Part print with two shaded views. Sizes in mm from the minimum x, y, z corner. A direction names the side the tool comes from. Round coordinates to 2 decimals unless told otherwise and drop trailing zeros. Write each loop counter-clockwise with the first axis right and the second up, starting at its lowest first coordinate (ties: lowest second). Pieces come first, ordered by that corner, then holes. Notation, with made-up numbers: (0, 78.5) -> (25, 78.5) arc R20 cw to (25, 108.5) -> close; hole circle Ø10 at (-27, 40). An arc over 180 degrees is marked (long way). Answer as CSV lines item,"result".
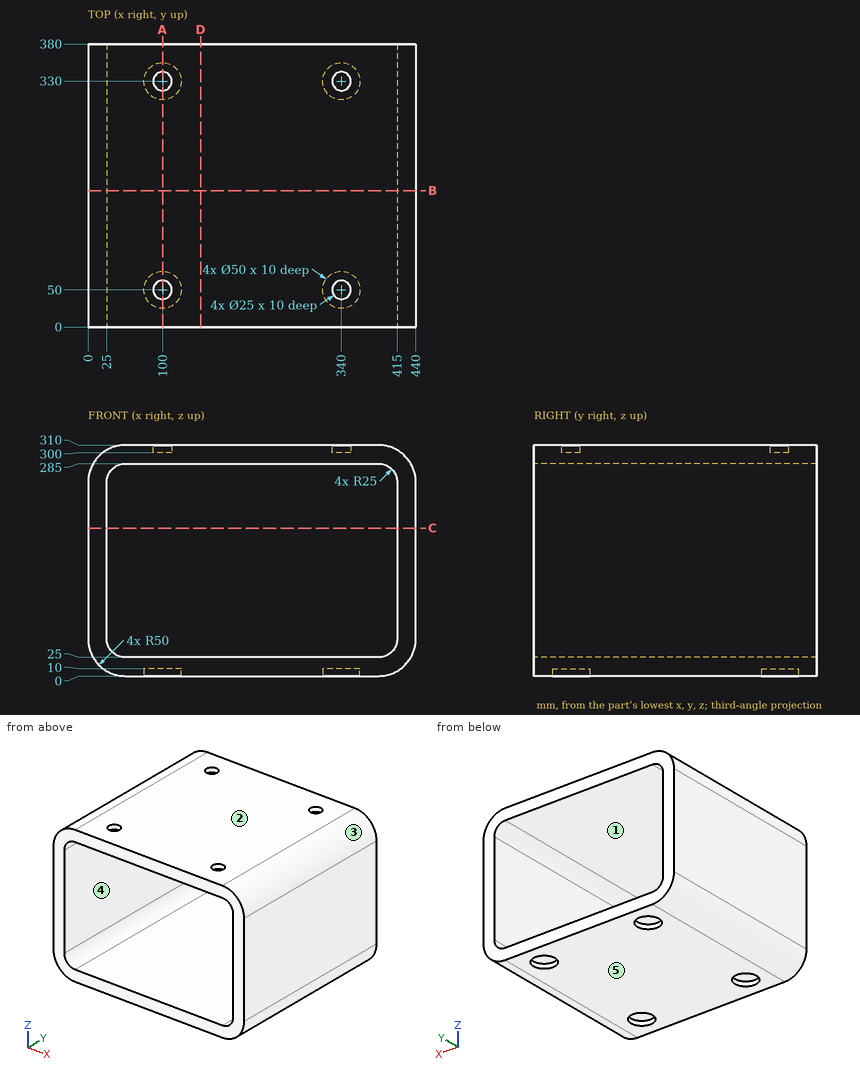
1. Cut at C-C, the plane z = 198.5. Write the cut outline in (x, y), then the cut area to 3 significant figures.
Results found:
outline,"(0, 0) -> (25, 0) -> (25, 380) -> (0, 380) -> close; (415, 0) -> (440, 0) -> (440, 380) -> (415, 380) -> close"
area,"19,000 mm2"
2. Mould opens along X. For the marked faces 3, 4 and 5 say: +X half, -X half, draft (parallel to the pull), parting line (faces both ways), or undercut.
Results found:
face 3,"+X half"
face 4,"undercut"
face 5,"draft"
3. Cut at D-D, the plane x = 151. Write the cut outline in (y, z).
Results found:
outline,"(0, 0) -> (380, 0) -> (380, 25) -> (0, 25) -> close; (0, 285) -> (380, 285) -> (380, 310) -> (0, 310) -> close"
4. Which spindle directions (+Z, -Z, +X, -X, +Y, -Y) get a long thin tool onto all of the face, cutting with end or side? Do the marked faces 1 and 2. Say none if no direction does.
Results found:
face 1,"+Y, -Y"
face 2,"+Z, +X, -X, +Y, -Y"
5. Probe line 1 along Y through (x, z) = (340, 2); line 2 along Y through (x, z) = (100, 302); line 3 along Z through (x, y) = (164, 176.5). List the from-to ranges inside material, lowest first.
Results found:
line 1,"y = 0 to 25, 75 to 305, 355 to 380"
line 2,"y = 0 to 37.5, 62.5 to 317.5, 342.5 to 380"
line 3,"z = 0 to 25, 285 to 310"
6. Cut at A-A, the plane x = 100. Write the cut outline in (y, z), then the cut area to 3 significant figures.
Results found:
outline,"(0, 0) -> (25, 0) -> (25, 10) -> (75, 10) -> (75, 0) -> (305, 0) -> (305, 10) -> (355, 10) -> (355, 0) -> (380, 0) -> (380, 25) -> (0, 25) -> close; (0, 285) -> (380, 285) -> (380, 310) -> (342.5, 310) -> (342.5, 300) -> (317.5, 300) -> (317.5, 310) -> (62.5, 310) -> (62.5, 300) -> (37.5, 300) -> (37.5, 310) -> (0, 310) -> close"
area,"17,500 mm2"
7. Cut at B-B, the plane y = 183. Write the cut outline in (x, z), then the cut area to 3 significant figures.
Results found:
outline,"(0, 50) arc R50 ccw to (50, 0) -> (390, 0) arc R50 ccw to (440, 50) -> (440, 260) arc R50 ccw to (390, 310) -> (50, 310) arc R50 ccw to (0, 260) -> close; hole (25, 50) arc R25 ccw to (50, 25) -> (390, 25) arc R25 ccw to (415, 50) -> (415, 260) arc R25 ccw to (390, 285) -> (50, 285) arc R25 ccw to (25, 260) -> close"
area,"33,400 mm2"
8. Drop flat-ended pins along their axis: pin 1 Ø15 at (x, y) = (340, 50) entering from -Z; pin 2 Ø12.5 at (x, y) = (337.5, 330) entering from +Z. Give the stop position or say it passes through.
Results found:
pin 1,"stops at z = 10"
pin 2,"stops at z = 300"
